Design review of the part built by this model. Coordinates are the model's own, in mm. A direction names the side the tool comes from. Round coordinates to 2 decimals unless told otherwise and drop trailing zeros. Order: outer loops, then holes, each group sorted by start corner. A loop starts at its lowest first (then second) coordinate and runs counter-clockwise, first axis right, second up. Notation, with made-up numbers: M 50,10 L 63,10 A22 ccw 63,45 Z; hole C 14.5,-5.5 d7. An arc over 180 degrees is marked long. Write item = value, one per line. Start each with the question number.
```python
from build123d import *

# Parameters (mm, degrees)
F2_DEPTH  = 8
F3_R      = 3.05
F4_DEPTH  = 45
F5_R      = 5.1
F6_DEPTH  = 6.1
F7_R      = 6
F8_DEPTH  = 10
F9_R      = 1.5
F10_DEPTH = 4.1915250807


with BuildPart() as f2:
    # F1 (on offset) → F2 (new body, symmetric)
    with BuildSketch(Plane.XZ.offset(-50)):
        Polygon((0, 55), (0, 10), (65, 10), (65, 55), (90, 55), (90, 65), (45, 65), (45, 55), align=None)
    extrude(amount=F2_DEPTH, both=True)

    # F3 (on face) → F4 (cut, through all)
    with BuildSketch(Plane.XY.offset(55)):
        with Locations((10, 50)):
            Circle(F3_R)
        with Locations((35, 50)):
            Circle(F3_R)
    extrude(amount=-F4_DEPTH, mode=Mode.SUBTRACT)

    # F5 (on face) → F6 (cut)
    with BuildSketch(Plane.XY.offset(55)):
        with Locations((10, 50)):
            Circle(F5_R)
        with Locations((35, 50)):
            Circle(F5_R)
    extrude(amount=-F6_DEPTH, mode=Mode.SUBTRACT)

    # F7 (on face) → F8 (cut, through all)
    with BuildSketch(Plane.XY.offset(65)):
        with Locations((80, 50)):
            Circle(F7_R)
    extrude(amount=-F8_DEPTH, mode=Mode.SUBTRACT)

    # F9 (on face) → F10 (cut, through all)
    with BuildSketch(Plane.YZ.offset(90)):
        with Locations((50, 60)):
            Circle(F9_R)
    extrude(amount=-F10_DEPTH, mode=Mode.SUBTRACT)


solid = f2.part
```
(1) Draft analysis for pull direction Y (two halves, no side actions). For faces 1 (the face through (34, 58, 38)), 2 (the face through (87.93, 48.89, 61.01)), 3 (the face through (23, 50, 55)), state which applies: pulls with the +Y half, pulls with the -Y half, needs draft (parallel to the pull), parting line crosses it, or undercut.
(2) Consider section C-C, the plane z = 57. Write out the cut boundary in (x, y), then the cut area to 3 significant figures.
(3) Consider section A-A, the plane x = 10. Write out the cut boundary in (y, z).
(4) Consider section B-B, the plane y = 50. State how many separate pieces and enclosed holes the cut face has, then the cut area to 3 significant figures.
(5) For faces 4 (the face through (9.9, 46.7, 48.9)), 5 (the face through (65, 50, 32)), 6 (the face through (45, 50, 60)), list the 3-axis set-ups (+Z, -Z, +X, -X, +Y, -Y) from which the entire face can be reached by the end or side of a thin tool; tool diameter is ignored.
(6) For line 1 along X through (y, z) = (51.75, 31.5); line 2 along X through (y, z) = (48.5, 47.5); line 3 along Y through (x, z) = (86, 60), list the stretches that pass through material, from the lowest coordinate up. Write a range as [from, to].
(7) Consider section D-D, the plane z = 29. Write out the cut boundary in (x, y).
(8) Insertion check: pin 1 (3 mm diameter, centred on x = 33, y = 51.5, fed in from +Z); pin 2 (5 mm diameter, centred on x = 10, y = 50, fed in from +Z); pin 3 (3 mm diameter, centred on y = 48.5, z = 61, fed in from -X); pin 4 (1 mm diameter, centred on y = 44, z = 21, fed in from +X). Each pin has a flat end and moves straight along its axis. Give the tip position at first contact, or say it passes through.
Completed:
q1.face_1 = pulls with the +Y half
q1.face_2 = undercut
q1.face_3 = needs draft
q2.outline = M 45,42 L 90,42 L 90,58 L 45,58 Z; hole C 80,50 d12
q2.area = 607 mm2
q3.outline = M 42,10 L 46.95,10 L 46.95,48.9 L 44.9,48.9 L 44.9,55 L 42,55 Z; M 53.05,10 L 58,10 L 58,55 L 55.1,55 L 55.1,48.9 L 53.05,48.9 Z
q4.separate_pieces = 5
q4.enclosed_holes = 0
q4.area = 2,640 mm2
q5.face_4 = +Z
q5.face_5 = -Z, +X, +Y, -Y
q5.face_6 = +Z, -X, +Y, -Y
q6.line_1 = [0, 7.5], [12.5, 32.5], [37.5, 65]
q6.line_2 = [0, 7.34], [12.66, 32.34], [37.66, 65]
q6.line_3 = [42, 48.5], [51.5, 58]
q7.outline = M 0,42 L 65,42 L 65,58 L 0,58 Z; hole C 10,50 d6.1; hole C 35,50 d6.1
q8.pin_1 = 48.9
q8.pin_2 = through
q8.pin_3 = 45
q8.pin_4 = 65
